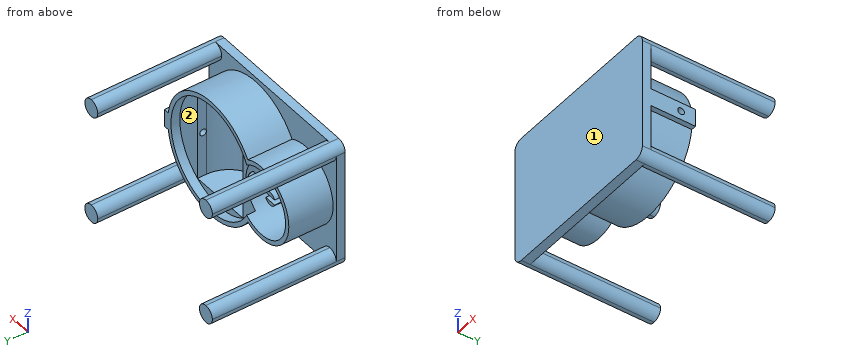
```python
from build123d import *

# Parameters (mm, degrees)
SKETCH1_W            = 39.5
SKETCH1_H            = 29
BOSS_EXTRUDE1_DEPTH  = 2
SKETCH2_R            = 13.5
SKETCH2_R_2          = 8.5
BOSS_EXTRUDE2_DEPTH  = 10
SKETCH3_R            = 12.5
CUT_EXTRUDE1_DEPTH   = 2
SKETCH4_R            = 7.5
CUT_EXTRUDE2_DEPTH   = 9
CUT_EXTRUDE3_START   = -10.3
CUT_EXTRUDE3_DEPTH   = 20.6
BOSS_EXTRUDE3_DEPTH  = 10
CUT_SWEEP1_START     = -214.913833497
CUT_SWEEP1_OUTLINE_R = 0.75
CUT_SWEEP1_DEPTH     = 22.537594322
BOSS_EXTRUDE4_DEPTH  = 7
SKETCH11_W           = 4
SKETCH11_H           = 4
BOSS_EXTRUDE5_DEPTH  = 28
FILLET1_R            = 2


# Read off the part's stored shape, not the designer's step: Cut-Extrude3, Cut-Sweep1
with BuildPart() as part:
    # Sketch1 → Boss-Extrude1 (new body)
    with BuildSketch(Plane(origin=(0, 0, 0), x_dir=(1, 0, 0), z_dir=(0, 1, 0))):
        with Locations((-212.126239175, -24.349172792)):
            Rectangle(SKETCH1_W, SKETCH1_H)
    extrude(amount=BOSS_EXTRUDE1_DEPTH)

    # Sketch2 → Boss-Extrude2 (add)
    with BuildSketch(Plane(origin=(0, 2, 0), x_dir=(1, 0, 0), z_dir=(0, 1, 0))):
        with Locations((-206.876239175, -24.349172792)):
            Circle(SKETCH2_R)
        with Locations((-222.376239175, -24.349172792)):
            Circle(SKETCH2_R_2)
    extrude(amount=BOSS_EXTRUDE2_DEPTH)

    # Sketch3 → Cut-Extrude1 (cut)
    with BuildSketch(Plane(origin=(0, 12, 0), x_dir=(1, 0, 0), z_dir=(0, 1, 0))):
        with Locations(Location((-206.876239175, -24.349172792, 0), (0, 0, 270))):
            Circle(SKETCH3_R)
    extrude(amount=-CUT_EXTRUDE1_DEPTH, mode=Mode.SUBTRACT)

    # Sketch4 → Cut-Extrude2 (cut)
    with BuildSketch(Plane(origin=(0, 12, 0), x_dir=(1, 0, 0), z_dir=(0, 1, 0))):
        with Locations(Location((-222.376239175, -24.349172792, 0), (0, 0, 270))):
            Circle(SKETCH4_R)
    extrude(amount=-CUT_EXTRUDE2_DEPTH, mode=Mode.SUBTRACT)

    # Cut-Extrude3 outline → Cut-Extrude3 (cut)
    with BuildSketch(Plane.XY.offset(24.349172792).offset(CUT_EXTRUDE3_START)):
        with BuildLine():
            ThreePointArc((-213.876239175, 8), (-206.876239175, 1), (-199.876239175, 8))
            Line((-199.876239175, 8), (-199.876239175, 10))
            Line((-199.876239175, 10), (-213.876239175, 10))
            Line((-213.876239175, 10), (-213.876239175, 8))
        make_face()
    extrude(amount=CUT_EXTRUDE3_DEPTH, mode=Mode.SUBTRACT)

    # Sketch7 → Boss-Extrude3 (add)
    with BuildSketch(Plane(origin=(0, 2, 0), x_dir=(1, 0, 0), z_dir=(0, 1, 0))):
        with BuildLine():
            Line((-192.376239175, -26.349172792), (-192.376239175, -24.349172792))
            Line((-192.376239175, -24.349172792), (-192.376239175, -22.349172792))
            Line((-192.376239175, -22.349172792), (-193.525209252, -22.349172792))
            ThreePointArc((-193.525209252, -22.349172792), (-193.413533207, -23.346402619), (-193.376239175, -24.349172792))
            ThreePointArc((-193.376239175, -24.349172792), (-193.413533207, -25.351942966), (-193.525209252, -26.349172792))
            Line((-193.525209252, -26.349172792), (-192.376239175, -26.349172792))
        make_face()
    extrude(amount=BOSS_EXTRUDE3_DEPTH)

    # Cut-Sweep1 outline → Cut-Sweep1 (cut)
    with BuildSketch(Plane.YZ.offset(CUT_SWEEP1_START)):
        with Locations((8.75, 24.349172792)):
            Circle(CUT_SWEEP1_OUTLINE_R)
    extrude(amount=CUT_SWEEP1_DEPTH, mode=Mode.SUBTRACT)

    # Sketch10 → Boss-Extrude4 (add)
    with BuildSketch(Plane(origin=(0, 3, 0), x_dir=(1, 0, 0), z_dir=(0, 1, 0))):
        with BuildLine():
            Line((-223.751011884, -23.749172792), (-222.376239175, -23.749172792))
            Line((-222.376239175, -23.749172792), (-221.001466467, -23.749172792))
            ThreePointArc((-221.001466467, -23.749172792), (-222.376239175, -22.849172792), (-223.751011884, -23.749172792))
        make_face()
        with BuildLine():
            Line((-221.001466467, -24.949172792), (-223.751011884, -24.949172792))
            ThreePointArc((-223.751011884, -24.949172792), (-222.376239175, -25.849172792), (-221.001466467, -24.949172792))
        make_face()
    extrude(amount=BOSS_EXTRUDE4_DEPTH)

    # Sketch11 → Boss-Extrude5 (add)
    with BuildSketch(Plane(origin=(0, 2, 0), x_dir=(1, 0, 0), z_dir=(0, 1, 0))):
        with Locations((-229.876239175, -36.849172792)):
            Rectangle(SKETCH11_W, SKETCH11_H)
        with Locations((-229.876239175, -11.849172792)):
            Rectangle(SKETCH11_W, SKETCH11_H)
        with Locations((-194.376239175, -36.849172792)):
            Rectangle(SKETCH11_W, SKETCH11_H)
        with Locations((-194.376239175, -11.849172792)):
            Rectangle(SKETCH11_W, SKETCH11_H)
    extrude(amount=BOSS_EXTRUDE5_DEPTH)

    # Fillet1
    fillet1_edges = [part.edges().sort_by_distance(p)[0] for p in [
        (-192.376239175, 16, 34.849172792),
        (-192.376239175, 15, 9.849172792),
        (-227.876239175, 16, 9.849172792),
        (-227.876239175, 16, 34.849172792),
        (-192.376239175, 16, 13.849172792),
        (-196.376239175, 16, 13.849172792),
        (-196.376239175, 16, 9.849172792),
        (-192.376239175, 15, 38.849172792),
        (-196.376239175, 16, 38.849172792),
        (-196.376239175, 16, 34.849172792),
        (-227.876239175, 16, 38.849172792),
        (-231.876239175, 15, 38.849172792),
        (-231.876239175, 16, 34.849172792),
        (-227.876239175, 16, 13.849172792),
        (-231.876239175, 16, 13.849172792),
        (-231.876239175, 15, 9.849172792),
    ]]
    fillet(fillet1_edges, radius=FILLET1_R - 0.0001)  # a hair under: the kernel refuses the full size


solid = part.part
```
Read the model definition and answer for the solid it produces. Units are mm, in the model's axes. Face numbers are marked on the shaded views. Give positions to 0.01 mm unless a question says otherwise; leave off trailing zeros. Write each loop counter-clockwise with the first axis right and the second up, starting at its lowest first coordinate (ties: lowest second). Pieces come first, ordered by that corner, then holes. Notation, with made-up numbers: (-23, -32.75) - (-1, -32.75) arc R19 ccw to (-1, -7.75) - close; hole circle Ø1 at (-26, 6.25). An arc over 180 degrees is marked (long way). Write item = value, one per line. Start each with the question number.
Item 1: Find section B-B (x = -202). Give the vertices of the cut face in (y, z).
Item 2: Each of these flat-tipped pins is pushed along its axis until it touches: P1, Ø0.6, axis at y = 9, z = 24, coming from the -X side; P2, Ø1, axis at x = -204, z = 22, coming from the +Y side; P3, Ø5, axis at x = -223, z = 28, coming from the +Y side; P4, Ø6, axis at x = -222, y = 26.5, coming from the +Z side. Where does it stop, or does it pass through?
Item 3: Find section C-C (z = 28). Give the vertices of the cut face in (x, y), then the cut area to 3 significant figures.
Item 4: Find the intervals of material crossed by probe 1 along Z at (x, y) = (-230, 12.5); probe 2 along X at (y, z) = (15.5, 11.75); probe 3 along X at (y, z) = (8.5, 29.25), in increasing order. Write a range as [from, to].
Item 5: Find section A-A (y = 13.5). State how many separate pieces and enclosed holes the cut face has, then the cut area to 3 significant figures.
Item 6: The mould has two halves that part along X. Classify the marked faces 1 and 2: +X half, -X half, draft (parallel to the pull), parting line (faces both ways), or undercut.
Response:
q1.outline = (0, 9.85) - (2, 9.85) - (2, 11.76) - (12, 11.76) - (12, 12.84) - (10, 12.84) - (10, 14.05) - (2.98, 14.05) - (2.98, 34.65) - (10, 34.65) - (10, 35.86) - (12, 35.86) - (12, 36.94) - (2, 36.94) - (2, 38.85) - (0, 38.85) - close
q2.P1 = -230.88
q2.P2 = 1.87
q2.P3 = 10
q2.P4 = through
q3.outline = (-231.88, 0) - (-192.38, 0) - (-192.38, 2) - (-193.88, 2) - (-193.88, 12) - (-194.92, 12) - (-194.92, 10) - (-199.88, 10) - (-199.88, 8) arc R7 cw to (-213.88, 8) - (-213.88, 10) - (-215.82, 10) - (-215.82, 3) - (-228.93, 3) - (-228.93, 12) - (-230.05, 12) - (-230.05, 2) - (-231.88, 2) - close
q3.area = 176 mm²
q4.probe_1 = [9.85, 13.85], [34.85, 38.85]
q4.probe_2 = [-231.87, -227.88], [-196.37, -192.38]
q4.probe_3 = [-229.32, -228.05], [-216.7, -213.88], [-199.88, -194.3]
q5.separate_pieces = 4
q5.enclosed_holes = 0
q5.area = 50.3 mm²
q6.face_1 = draft
q6.face_2 = undercut
